Part model, mm, in its own coordinate system. Round coordinates to 2 decimals unless told otherwise and drop trailing zeros. Loops run counter-clockwise (first coordinate to the right, second up) from the corner with the lowest first, then second, coordinate; pieces in that order, holes last.
1) Band-saw the part on A-A, the plane x = -81. Write the cut outline in (y, z).
2) Drop flat-ended pins along their axis: P1, Ø3, axis at x = -83.5, z = 2, coming from the +Y side; P2, Ø2.5, axis at x = -41.5, z = 2.5, coming from the -Y side; P3, Ø2, axis at y = -16.5, z = 3.5, coming from the +X side. Give the stop position or say it passes through.
3) Probe line 1 (Y direction, x = -1, z = 4.45). List the from-to ranges inside material, lowest first.
from build123d import *

# Parameters (mm, degrees)
ESQUISSE1_W        = 90
ESQUISSE1_H        = 90
BOSS_EXTRU_1_DEPTH = 5
ESQUISSE2_W        = 5
ESQUISSE2_H        = 18
BOSS_EXTRU_2_DEPTH = 5
ESQUISSE3_W        = 18
ESQUISSE3_H        = 5
BOSS_EXTRU_3_DEPTH = 5


with BuildPart() as part:
    # Esquisse1 → Boss.-Extru.1 (new body)
    with BuildSketch(Plane.XY):
        with Locations((-45, -45)):
            Rectangle(ESQUISSE1_W, ESQUISSE1_H)
    extrude(amount=BOSS_EXTRU_1_DEPTH)

    # Esquisse2 → Boss.-Extru.2 (add)
    with BuildSketch(Plane(origin=(0, 0, 0), x_dir=(-1, 0, 0), z_dir=(0, 0, -1))):
        with Locations((-2.5, -27)):
            Rectangle(ESQUISSE2_W, ESQUISSE2_H)
        with Locations((-2.5, -63)):
            Rectangle(ESQUISSE2_W, ESQUISSE2_H)
        with Locations((92.5, -63)):
            Rectangle(ESQUISSE2_W, ESQUISSE2_H)
        with Locations((92.5, -27)):
            Rectangle(ESQUISSE2_W, ESQUISSE2_H)
    extrude(amount=-BOSS_EXTRU_2_DEPTH)

    # Esquisse3 → Boss.-Extru.3 (add)
    with BuildSketch(Plane(origin=(0, 0, 0), x_dir=(-1, 0, 0), z_dir=(0, 0, -1))):
        with Locations((27, 2.5)):
            Rectangle(ESQUISSE3_W, ESQUISSE3_H)
        with Locations((63, 2.5)):
            Rectangle(ESQUISSE3_W, ESQUISSE3_H)
        with Locations((63, -92.5)):
            Rectangle(ESQUISSE3_W, ESQUISSE3_H)
        with Locations((27, -92.5)):
            Rectangle(ESQUISSE3_W, ESQUISSE3_H)
    extrude(amount=-BOSS_EXTRU_3_DEPTH)


solid = part.part
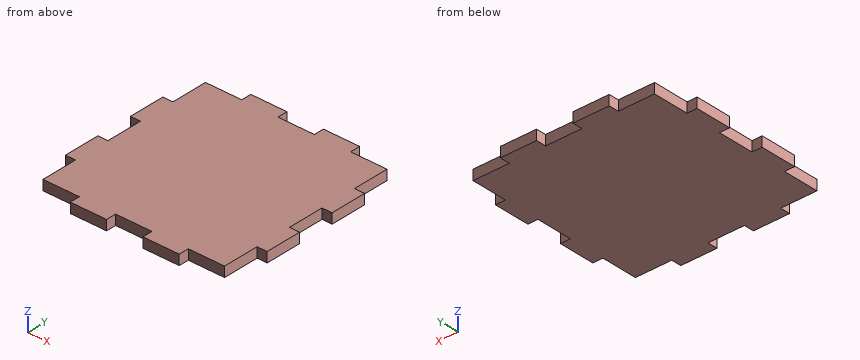
Reported:
1. outline: (-90, 0) - (0, 0) - (0, 5) - (-90, 5) - close
2. P1: stops at y = 0
2. P2: stops at y = -90
2. P3: stops at x = 0
3. line 1: y = -90 to 0
